Here's the drawing with two shaded views (mm, measured from the low corner). I have some questions. Round coordinates to 2 decimals unless told otherwise and drop trailing zeros. Loops run counter-clockwise (first coordinate to the right, second up) from the corner with the lowest first, then second, coordinate; pieces in that order, holes last.
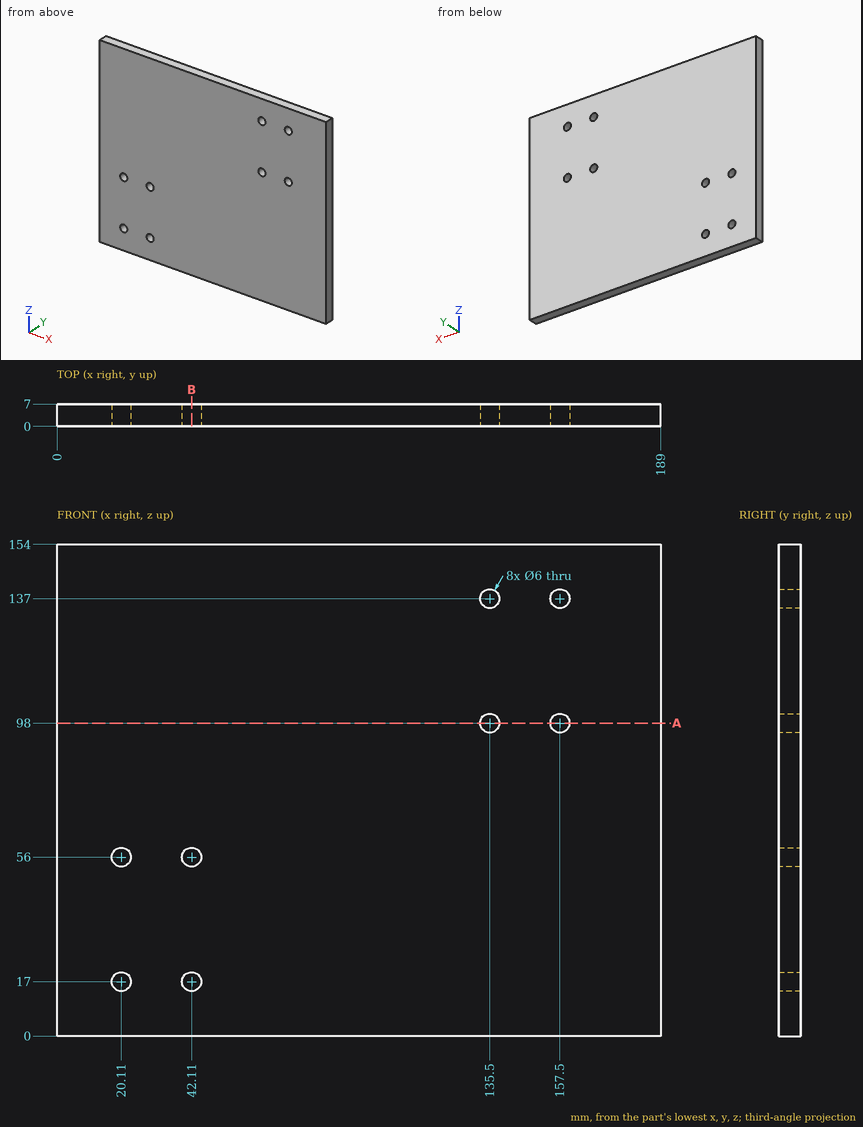
Item 1: Will this pin go through, and if not, where does the flat tip stop? pin 1 (5.5 mm diameter, centred on x = 42.11, z = 56, fed in from -Y).
Results list:
pin 1: passes through
Item 2: If I drill on line 1 along X through (y, z) = (3.25, 56); line 2 along Z through (x, y) = (157.5, 2.25); line 3 along X through (y, z) = (3.75, 98), over which ranges is the centre line in solid material (lowest first)?
Results list:
line 1: x = 0 to 17.11, 23.11 to 39.11, 45.11 to 189
line 2: z = 0 to 95, 101 to 134, 140 to 154
line 3: x = 0 to 132.5, 138.5 to 154.5, 160.5 to 189
Item 3: If we section it at A-A, the plane z = 98: Please give me the cut outline in (x, y), then the cut area to 3 significant figures.
Results list:
outline: (0, 0) - (132.5, 0) - (132.5, 7) - (0, 7) - close; (138.5, 0) - (154.5, 0) - (154.5, 7) - (138.5, 7) - close; (160.5, 0) - (189, 0) - (189, 7) - (160.5, 7) - close
area: 1,240 mm2
Item 4: If we section it at B-B, the plane x = 42.11: Please give me the cut outline in (y, z), then the cut area to 3 significant figures.
Results list:
outline: (0, 0) - (7, 0) - (7, 14) - (0, 14) - close; (0, 20) - (7, 20) - (7, 53) - (0, 53) - close; (0, 59) - (7, 59) - (7, 154) - (0, 154) - close
area: 994 mm2
